```python
from build123d import *

# Parameters (mm, degrees)
SKETCH2_W           = 76.2
SKETCH2_H           = 63.5
BOSS_EXTRUDE1_DEPTH = 44.45
SKETCH5_W           = 25.4
SKETCH5_H           = 50.8
CUT_EXTRUDE3_DEPTH  = 94.756626432
CUT_EXTRUDE4_DEPTH  = 44.45
CUT_EXTRUDE5_DEPTH  = 67.599361859
SKETCH7_R           = 3.175
CUT_EXTRUDE6_DEPTH  = 44.45
SKETCH8_R           = 3.81
CUT_EXTRUDE7_DEPTH  = 67.599361859
FILLET3_R           = 2.54


with BuildPart() as part:
    # Sketch2 → Boss-Extrude1 (new body)
    with BuildSketch(Plane.XY):
        Rectangle(SKETCH2_W, SKETCH2_H)
    extrude(amount=BOSS_EXTRUDE1_DEPTH)

    # Sketch5 → Cut-Extrude3 (cut, through all)
    with BuildSketch(Plane(origin=(38.1, 0, 0), x_dir=(0, 0, -1), z_dir=(1, 0, 0))):
        with Locations((-22.225, 6.35)):
            Rectangle(SKETCH5_W, SKETCH5_H)
    extrude(amount=-CUT_EXTRUDE3_DEPTH, mode=Mode.SUBTRACT)

    # Sketch3 → Cut-Extrude4 (cut)
    with BuildSketch(Plane.XY.offset(44.45)):
        Polygon((-38.1, -31.75), (0, 31.75), (-38.1, 31.75), align=None)
    extrude(amount=-CUT_EXTRUDE4_DEPTH, mode=Mode.SUBTRACT)

    # Sketch6 → Cut-Extrude5 (cut, through all)
    with BuildSketch(Plane.XY.offset(44.45)):
        Polygon((0, 31.75), (38.1, -31.75), (38.1, 31.75), align=None)
    extrude(amount=-CUT_EXTRUDE5_DEPTH, mode=Mode.SUBTRACT)

    # Sketch7 → Cut-Extrude6 (cut)
    with BuildSketch(Plane(origin=(0, -19.05, 0), x_dir=(1, 0, 0), z_dir=(0, 1, 0))):
        with Locations(Location((-19.05, -15.737033212, 0), (0, 0, 180))):
            Circle(SKETCH7_R)
        with Locations(Location((19.05, -15.737033212, 0), (0, 0, 270))):
            Circle(SKETCH7_R)
        with Locations(Location((19.05, -28.437033212, 0), (0, 0, 180))):
            Circle(SKETCH7_R)
        with Locations(Location((-19.05, -28.437033212, 0), (0, 0, 270))):
            Circle(SKETCH7_R)
    extrude(amount=-CUT_EXTRUDE6_DEPTH, mode=Mode.SUBTRACT)

    # Sketch8 → Cut-Extrude7 (cut, through all)
    with BuildSketch(Plane.XY.offset(44.45)):
        with Locations((0, 12.7)):
            Circle(SKETCH8_R)
    extrude(amount=-CUT_EXTRUDE7_DEPTH, mode=Mode.SUBTRACT)

    # Fillet3
    fillet3_edges = [part.edges().sort_by_distance(p)[0] for p in [
        (0, 31.75, 4.7625),
        (0, 31.75, 39.6875),
        (38.1, -31.75, 22.225),
        (-38.1, -31.75, 22.225),
    ]]
    fillet(fillet3_edges, radius=FILLET3_R)


solid = part.part
```
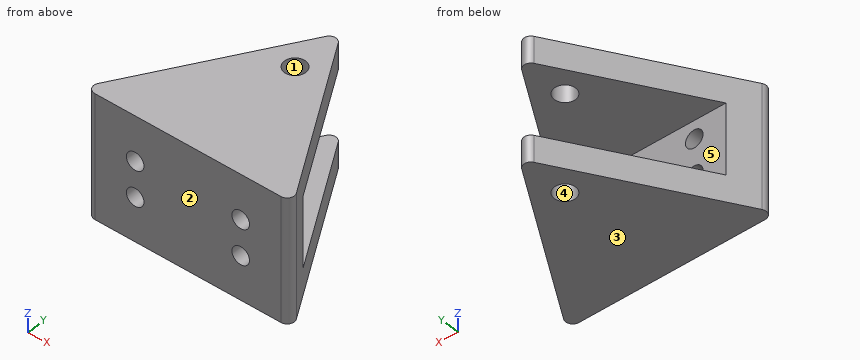
Source: CAD feature listing. Evaluate the final solid. Frame: model axes, mm. Face numbers are marked on the shaded views. A direction names the side the tool comes from. Give positions to 0.01 mm unless a question says otherwise; leave off trailing zeros. Order: outer loops, then holes, each group sorted by start corner. A loop starts at its lowest first (then second) coordinate and runs counter-clockwise, first axis right, second up. Notation, with made-up numbers: (-25, 6.25) -> (27, 6.25) arc R13 ccw to (27, 12.25) -> close; hole circle Ø1 at (84.5, -6.75). An arc over 180 degrees is marked (long way). Use a Markdown table: item, result.
Q1. Section A-A (z = 40). Return the cut outline in (x, y).
A:
| item | result |
|---|---|
| outline | (-35.79, -27.9) arc R2.54 ccw to (-33.61, -31.75) -> (33.61, -31.75) arc R2.54 ccw to (35.79, -27.9) -> (2.18, 28.12) arc R2.54 ccw to (-2.18, 28.12) -> close; hole circle Ø7.62 at (0, 12.7) |
Q2. Section B-B (y = -5). Return the cut outline in (x, z) (3 decimals).
A:
| item | result |
|---|---|
| outline | (-22.05, 0) -> (22.05, 0) -> (22.05, 9.525) -> (-22.05, 9.525) -> close; (-22.05, 34.925) -> (22.05, 34.925) -> (22.05, 44.45) -> (-22.05, 44.45) -> close |
Q3. First-contact query: P1, Ø1, axis at x = 1, z = 14.5, coming from the +Y side; P2, Ø8, axis at x = 26, z = 20.5, coming from the +Y side. Flat tips, straight axial feed; report the tip coordinate or a pass-through.
A:
| item | result |
|---|---|
| P1 | y = -19.05 |
| P2 | y = -19.05 |
Q4. Section D-D (z = 33). Return the cut outline in (x, y).
A:
| item | result |
|---|---|
| outline | (-35.79, -27.9) arc R2.54 ccw to (-33.61, -31.75) -> (33.61, -31.75) arc R2.54 ccw to (35.79, -27.9) -> (30.48, -19.05) -> (-30.48, -19.05) -> close |
Q5. Access query for the marked faces 4 and 5. Directions: +Z, -Z, +X, -X, +Y, -Y. A direction counts if a zero-diameter tool reaches every point of the face in a straight line with its end or side. Return the directions, or none.
A:
| item | result |
|---|---|
| face 4 | +Z, -Z |
| face 5 | +X, -X, +Y |
Q6. Pull-direction query (Y, two-part tool) for the marked faces 1, 2 and 3; classes: +Y half, -Y half, draft (parallel to the pull), parting line (faces both ways), or undercut.
A:
| item | result |
|---|---|
| face 1 | undercut |
| face 2 | -Y half |
| face 3 | draft |
Q7. Material intervals for line 1 (Y direction, x = 0, z = 39); line 2 (Z direction, x = 5, y = -9.5) (3 decimals); line 3 (Y direction, x = -5.5, z = 34), sorted ascending. Write a range as [from, to].
A:
| item | result |
|---|---|
| line 1 | [-31.75, 8.89], [16.51, 29.35] |
| line 2 | [0, 9.525], [34.925, 44.45] |
| line 3 | [-31.75, -19.05] |
Q8. Section C-C (x = 19.05). Return the cut outline in (y, z) (3 decimals).
A:
| item | result |
|---|---|
| outline | (-31.75, 0) -> (0, 0) -> (0, 9.525) -> (-19.05, 9.525) -> (-19.05, 12.562) -> (-31.75, 12.562) -> close; (-31.75, 18.912) -> (-19.05, 18.912) -> (-19.05, 25.262) -> (-31.75, 25.262) -> close; (-31.75, 31.612) -> (-19.05, 31.612) -> (-19.05, 34.925) -> (0, 34.925) -> (0, 44.45) -> (-31.75, 44.45) -> close |
